Can you work these out from the drawing? Everything is in mm from the part's minimum corner. Give positions to 0.01 mm unless a question says otherwise; leave off trailing zeros. Order: outer loops, then holes, each group sorted by start corner. A loop starts at its lowest first (then second) coordinate and runs counter-clockwise, first axis right, second up. Notation, with made-up numbers: (44, 66.25) -> (93, 66.25) arc R26 cw to (93, 90.25) -> close; hole circle Ø4 at (89.25, 64.25). An arc over 180 degrees is marked (long way). One line per item, written item: value.
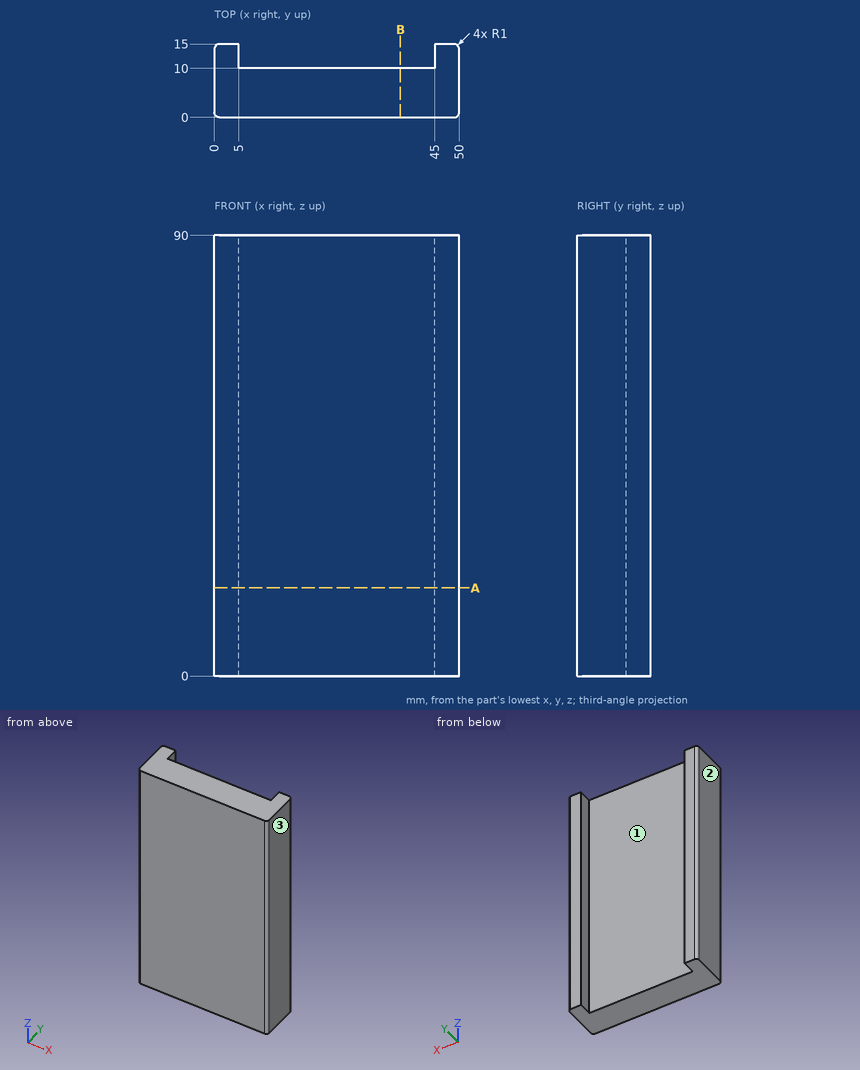
1) Suppose I cut it at B-B, the plane x = 38. Write out the boundary of the cut face in (y, z).
Answer below:
outline: (0, 0) -> (10, 0) -> (10, 90) -> (0, 90) -> close
2) For P1, Ø2, axis at x = 23, z = 76, coming from the +Y side, with a flat end and sliding along its axis, tell me the tip position at first contact or that it passes through.
Answer below:
P1: stops at y = 10
3) If I drill on line 1 along X through (y, z) = (10.75, 28.5); line 2 along Y through (x, z) = (40, 61.5), over which ranges is the centre line in solid material (lowest first)?
Answer below:
line 1: x = 0 to 5, 45 to 50
line 2: y = 0 to 10
4) Suppose I cut it at A-A, the plane z = 18. Write out the boundary of the cut face in (x, y).
Answer below:
outline: (0, 1) arc R1 ccw to (1, 0) -> (49, 0) arc R1 ccw to (50, 1) -> (50, 14) arc R1 ccw to (49, 15) -> (45, 15) -> (45, 10) -> (5, 10) -> (5, 15) -> (1, 15) arc R1 ccw to (0, 14) -> close
5) We'd pull the mould along X, two halves only. Please class the marked faces 1, 2 and 3: +X half, -X half, draft (parallel to the pull), parting line (faces both ways), or undercut.
Answer below:
face 1: undercut
face 2: -X half
face 3: +X half
